Autodesk Inventor part; units mm, degrees
ref_plane "Plan YZ" through (0, 0, 0) normal (1, 0, 0) x (0, 1, 0)
ref_plane "Plan XZ" through (0, 0, 0) normal (0, 1, 0) x (-1, 0, 0)
ref_plane "Plan XY" through (0, 0, 0) normal (0, 0, 1) x (1, 0, 0)
sketch "Esquisse1" plane through (0, 0, 0) normal (0, 0, 1) x (1, 0, 0)
  circle A0 centre (0, 0) radius 1.425
  dimension "d0" = 2.85
extrude "Extrusion1" add sketch "Esquisse1" along normal blind 5
sketch "Esquisse6" plane through (0, 0, 5) normal (0, 0, 1) x (1, 0, 0)
  line L0 (-4.8497, 0) -> (4.8497, 0) construction
  line L1 (0, -4.2) -> (0, 4.2) construction
  line L2 (-1.7321, -3) -> (-3.4641, 0)
  line L3 (-3.4641, 0) -> (-1.7321, 3)
  line L4 (-1.7321, 3) -> (0, 3)
  line L5 (-1.7321, -3) -> (0, -3)
  line L6 (1.7321, -3) -> (3.4641, 0)
  line L7 (3.4641, 0) -> (1.7321, 3)
  line L8 (1.7321, 3) -> (0, 3)
  line L9 (1.7321, -3) -> (0, -3)
  point P0 (0, 0)
  dimension "d4" = 6
  dimension "d8" = 120
  dimension "d10" = 6
extrude "Extrusion2" add sketch "Esquisse6" along normal blind 6
sketch "Esquisse7" plane through (0, 0, 11) normal (0, 0, 1) x (1, 0, 0)
  circle A0 centre (0, 0) radius 1.425
hole "Perçage1" at (0, 0, 11) direction (0, 0, -1) diameter 2.459 depth 5 tip angle 118
thread "Filetage1"
properties part number "Entretoise_M3x6" material "."
For this review, take the finished solid that the model builds, in its own axes (mm). A direction names the side the tool comes from. Give positions to 0.01 mm unless a question says otherwise; leave off trailing zeros. Order: outer loops, then holes, each group sorted by start corner. A loop starts at its lowest first (then second) coordinate and runs counter-clockwise, first axis right, second up. Notation, with made-up numbers: (44, 22.25) -> (84, 22.25) arc R21 ccw to (84, 48.25) -> close; hole circle Ø10 at (83.25, 65.25). An arc over 180 degrees is marked (long way). Write item = value, one per line.
1) We need section B-B, the plane z = 2.25. Give the boundary of the cut face in (x, y) (3 decimals), and give its area (3 significant figures).
Findings:
outline = circle Ø2.85 at (0, 0)
area = 6.38 mm^2
2) Insertion check: pin 1 (2 mm diameter, centred on x = 0, y = 0, fed in from +Z); pin 2 (1 mm diameter, centred on x = -2.5, y = 2.5, fed in from -Z); pin 3 (1.5 mm diameter, centred on x = 1.5, z = 1.5, fed in from -Y); pin 4 (1 mm diameter, centred on x = -2, z = 3.5, fed in from +Y). Each pin has a flat end and moves straight along its axis. Give the tip position at first contact, or say it passes through.
Findings:
pin_1 = 5.86
pin_2 = 5
pin_3 = -1.21
pin_4 = through
3) To check wall thickness, follow L1, parallel to Y at x = 0, z = 7.5; L2, parallel to Y at x = -0.75, z = 10; L3, parallel to Z at x = -1, y = 2.7. State the ranges of each line that lie inside material, in increasing order. Write a range as from..to.
Findings:
L1 = -3..-1.23, 1.23..3
L2 = -3..-0.97, 0.97..3
L3 = 5..11
4) We need section A-A, the plane z = 9.25. Give the boundary of the cut face in (x, y), and give its area (3 significant figures).
Findings:
outline = (-3.46, 0) -> (-1.73, -3) -> (1.73, -3) -> (3.46, 0) -> (1.73, 3) -> (-1.73, 3) -> close; hole circle Ø2.46 at (0, 0)
area = 26.4 mm^2
5) Draft analysis for pull direction X (two halves, no side actions). For faces 1 (the face through (1.5, 0, 11)), 2 (the face through (-2.6, -1.5, 8)), 3 (the face through (0.748, 0.976, 8.465)), 4 (the face through (2.6, 1.5, 8)), state which applies: pulls with the +X half, pulls with the -X half, needs draft (parallel to the pull), parting line crosses it, or undercut.
Findings:
face_1 = needs draft
face_2 = pulls with the -X half
face_3 = undercut
face_4 = pulls with the +X half
6) We need section C-C, the plane y = 1.95. Give the boundary of the cut face in (x, z).
Findings:
outline = (-2.34, 5) -> (2.34, 5) -> (2.34, 11) -> (-2.34, 11) -> close
7) For faces 5 (the face through (-2.6, 1.5, 8)), 6 (the face through (-1.13, 0.87, 2.46)), list the 3-axis set-ups (+Z, -Z, +X, -X, +Y, -Y) from which the entire face can be reached by the end or side of a thin tool; tool diameter is ignored.
Findings:
face_5 = +Z, -Z, -X, +Y
face_6 = -Z
